Work out the finished part from the listing and answer in its coordinate system (mm). Face numbers are marked on the shaded views. A direction names the side the tool comes from. Round coordinates to 2 decimals unless told otherwise and drop trailing zeros. Write each loop counter-clockwise with the first axis right and the second up, starting at its lowest first coordinate (ties: lowest second). Pieces come first, ordered by that corner, then holes. Notation, with made-up numbers: M 32,12.25 L 72,12.25 A28 ccw 72,32.25 Z; hole C 80,33 d11. An arc over 180 degrees is marked long. Answer in a Markdown table with one row per item.
```python
from build123d import *

# Parameters (mm, degrees)
SKETCH1_3_W                     = 6.35
SKETCH1_3_H                     = 63.5
BOSS_EXTRUDE1_DEPTH             = 63.5
SKETCH1_W                       = 50.8
SKETCH1_H                       = 63.5
BOSS_EXTRUDE2_DEPTH             = 6.35
SKETCH1_6_W                     = 6.35
SKETCH1_6_H                     = 63.5
BOSS_EXTRUDE3_DEPTH             = 63.5
SKETCH2_R                       = 14.2875
CUT_EXTRUDE1_DEPTH              = 96.25
F_43_0_089_DIAMETER_HOLE1_D     = 2.2606
F_43_0_089_DIAMETER_HOLE1_DEPTH = 25.4
F_43_0_089_DIAMETER_HOLE1_TIP   = 0.679152758
F_10_32_TAPPED_HOLE1_D          = 4.0386
F_10_32_TAPPED_HOLE1_DEPTH      = 6.35


with BuildPart() as part:
    # Sketch1<3> → Boss-Extrude1 (new body)
    with BuildSketch(Plane(origin=(0, 0, 0), x_dir=(1, 0, 0), z_dir=(0, 1, 0))):
        with Locations((28.575, 0)):
            Rectangle(SKETCH1_3_W, SKETCH1_3_H)
    extrude(amount=BOSS_EXTRUDE1_DEPTH)

    # Sketch1 → Boss-Extrude2 (add)
    with BuildSketch(Plane(origin=(0, 0, 0), x_dir=(1, 0, 0), z_dir=(0, 1, 0))):
        Rectangle(SKETCH1_W, SKETCH1_H)
    extrude(amount=BOSS_EXTRUDE2_DEPTH)

    # Sketch1<6> → Boss-Extrude3 (add)
    with BuildSketch(Plane(origin=(0, 0, 0), x_dir=(1, 0, 0), z_dir=(0, 1, 0))):
        with Locations((-28.575, 0)):
            Rectangle(SKETCH1_6_W, SKETCH1_6_H)
    extrude(amount=BOSS_EXTRUDE3_DEPTH)

    # Sketch2 → Cut-Extrude1 (cut, through all)
    with BuildSketch(Plane(origin=(31.75, 0, 0), x_dir=(0, 0, -1), z_dir=(1, 0, 0))):
        with Locations((0, 31.75)):
            Circle(SKETCH2_R)
    extrude(amount=-CUT_EXTRUDE1_DEPTH, mode=Mode.SUBTRACT)

    # #43 (0.089) Diameter Hole1
    with Locations(Plane.ZY.offset(31.75)):
        with Locations((-19.05, 50.8), (19.05, 50.8), (19.05, 12.7), (-19.05, 12.7)):
            Hole(F_43_0_089_DIAMETER_HOLE1_D / 2, depth=F_43_0_089_DIAMETER_HOLE1_DEPTH)
            with Locations((0, 0, -(F_43_0_089_DIAMETER_HOLE1_DEPTH + F_43_0_089_DIAMETER_HOLE1_TIP / 2))):  # 118° drill point
                Cone(0, F_43_0_089_DIAMETER_HOLE1_D / 2, F_43_0_089_DIAMETER_HOLE1_TIP, mode=Mode.SUBTRACT)

    # #10-32 Tapped Hole1
    with Locations(Plane(origin=(31.75, 0, 0), x_dir=(0, 0, -1), z_dir=(1, 0, 0))):
        with Locations((-23.495, 55.245), (23.495, 55.245), (23.495, 8.255), (-23.495, 8.255)):
            Hole(F_10_32_TAPPED_HOLE1_D / 2, depth=F_10_32_TAPPED_HOLE1_DEPTH)


solid = part.part
```
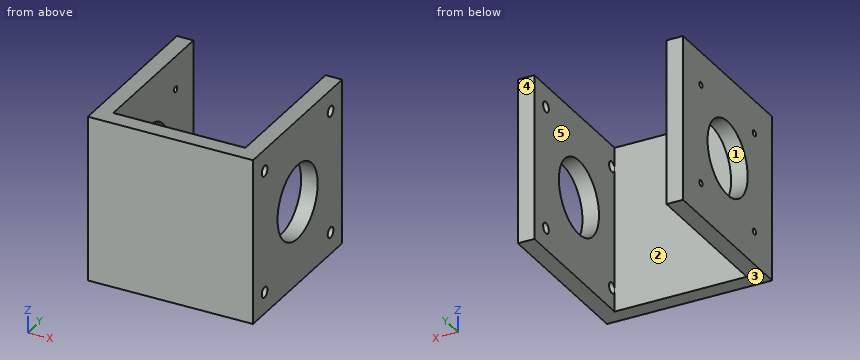
1. The part is cut by section B-B (y = 12.7). Determine the outline of the cut face in (x, z), plus the area to 3 significant figures.
Calculated:
| item | result |
|---|---|
| outline | M -31.75,-31.75 L -25.4,-31.75 L -25.4,-20.18 L -31.75,-20.18 Z; M -31.75,-17.92 L -25.4,-17.92 L -25.4,17.92 L -31.75,17.92 Z; M -31.75,20.18 L -25.4,20.18 L -25.4,31.75 L -31.75,31.75 Z; M 25.4,-31.75 L 31.75,-31.75 L 31.75,31.75 L 25.4,31.75 Z |
| area | 778 mm² |
2. The part is cut by section D-D (z = -19.05). Determine the outline of the cut face in (x, y).
Calculated:
| item | result |
|---|---|
| outline | M -31.75,0 L 31.75,0 L 31.75,63.5 L 25.4,63.5 L 25.4,6.35 L -25.4,6.35 L -25.4,11.57 L -31.75,11.57 Z; M -31.75,13.83 L -25.4,13.83 L -25.4,49.67 L -31.75,49.67 Z; M -31.75,51.93 L -25.4,51.93 L -25.4,63.5 L -31.75,63.5 Z |
3. A tool of negligible diameter and unlimited length cuts with its end or side. For the marked faces 4 and 5, from which of +Z, -Z, +X, -X, +Y, -Y can it reach the whole face along a straight path? Write none if from no direction.
Calculated:
| item | result |
|---|---|
| face 4 | +Z, -Z, +X, -X, +Y |
| face 5 | +Z, -Z, +Y |
4. Consider line 1 along Y through (x, z) = (-29.25, 19.05); line 2 along X through (y, z) = (54.5, -27.5); line 3 along Y through (x, z) = (-26.75, 0). Determine where each line is inside the solid, lowest interval first. Write a range as from..to.
Calculated:
| item | result |
|---|---|
| line 1 | y = 0..11.57, 13.83..49.67, 51.93..63.5 |
| line 2 | x = -31.75..-25.4, 25.4..31.75 |
| line 3 | y = 0..17.46, 46.04..63.5 |
5. Determine the mould class of the marked faces 1, 2 and 3 for opening direction Y: released by +Y, released by -Y, zero draft, split by the parting line, or undercut.
Calculated:
| item | result |
|---|---|
| face 1 | undercut |
| face 2 | released by +Y |
| face 3 | zero draft |
6. The part is cut by section A-A (z = 0). Determine the outline of the cut face in (x, y), plus the area to 3 significant figures.
Calculated:
| item | result |
|---|---|
| outline | M -31.75,0 L 31.75,0 L 31.75,17.46 L 25.4,17.46 L 25.4,6.35 L -25.4,6.35 L -25.4,17.46 L -31.75,17.46 Z; M -31.75,46.04 L -25.4,46.04 L -25.4,63.5 L -31.75,63.5 Z; M 25.4,46.04 L 31.75,46.04 L 31.75,63.5 L 25.4,63.5 Z |
| area | 766 mm² |
7. The part is cut by section C-C (y = 59.5). Determine the outline of the cut face in (x, z), plus the area to 3 significant figures.
Calculated:
| item | result |
|---|---|
| outline | M -31.75,-31.75 L -25.4,-31.75 L -25.4,31.75 L -31.75,31.75 Z; M 25.4,-31.75 L 31.75,-31.75 L 31.75,31.75 L 25.4,31.75 Z |
| area | 806 mm² |
8. Given pin 1 (1.5 mm diameter, centred on x = 21.5, z = -21.5, fed in from +Y); pin 2 (3.5 mm diameter, centred on y = 55.245, z = 23.495, fed in from +X); pin 3 (2 mm diameter, centred on y = 50.8, z = 19.05, fed in from -X), each flat-ended and moving along its own axis, determine where each tip first touches the part or whether it passes through.
Calculated:
| item | result |
|---|---|
| pin 1 | stops at y = 6.35 |
| pin 2 | stops at x = -25.4 |
| pin 3 | stops at x = 25.4 |
